```python
from build123d import *

# Parameters (mm, degrees)
F0_R     = 12.7
F1_DEPTH = 127
F2_R     = 3.175
F3_W     = 3.429
F3_H     = 3.429
F4_DEPTH = 127.001


with BuildPart() as f1:
    # F0 (on Top) → F1 (new body)
    with BuildSketch(Plane.XY):
        Circle(F0_R)
    extrude(amount=F1_DEPTH)

    # F2
    f2_edges = [f1.edges().sort_by_distance(p)[0] for p in [
        (-12.7, 0, 127),
    ]]
    fillet(f2_edges, radius=F2_R)

    # F3 (on face) → F4 (cut, through all)
    with BuildSketch(Plane.XY.offset(127)):
        Rectangle(F3_W, F3_H)
    extrude(amount=-F4_DEPTH, mode=Mode.SUBTRACT)


solid = f1.part
```
Geometry check sheet. Reference: the model listing, model coordinates, mm. A direction names the side the tool comes from. Give positions to 0.01 mm unless a question says otherwise; leave off trailing zeros. Write each loop counter-clockwise with the first axis right and the second up, starting at its lowest first coordinate (ties: lowest second). Pieces come first, ordered by that corner, then holes.
1) Gauge pin test, flat ends, axial feed: pin 1 (5 mm diameter, centred on x = -4, z = 93.5, fed in from -Y); pin 2 (8 mm diameter, centred on y = -5.5, z = 65.5, fed in from +X); pin 3 (1.5 mm diameter, centred on x = -0.5, y = 0, fed in from +Z); pin 4 (1 mm diameter, centred on x = -8.5, z = 25, fed in from +Y). Record the tip position at first contact, or that the pin passes through.
2) Access from +Z, -Z, +X, -X, +Y, -Y to the whole of each face (thin tool, end or side, straight path). Record for faces 5 (the flat face through (-1.714, 0, 64)), 6 (the flat face through (3, 0, 0)).
3) Material ranges on L1, parallel to Y at x = 0.75, z = 68; L2, parallel to Y at x = -1.25, z = 48.5; L3, parallel to X at y = 6, z = 113, recorded low to high.
4) Section check C-C, the plane z = 41.5. Record the boundary of the cut face in (x, y), and give its area (3 significant figures).
5) Release check for a two-part mould opening along X. For faces 1 (the flat face through (2, 0, 127)), 2 (the flat face through (0, 1.714, 64)), 3 (the cylindrical face through (-2.75, -12.4, 61.05)), 4 (the flat face through (1.714, 0, 64)) record: pulls with the +X half, pulls with the -X half, needs draft (parallel to the pull), parting line crosses it, or undercut.
Computed:
1. pin 1: stops at y = -12.61
1. pin 2: stops at x = 12.61
1. pin 3: passes through
1. pin 4: stops at y = 9.86
2. face 5: +Z, -Z
2. face 6: -Z, +X, -X, +Y, -Y
3. L1: y = -12.68 to -1.71, 1.71 to 12.68
3. L2: y = -12.64 to -1.71, 1.71 to 12.64
3. L3: x = -11.19 to 11.19
4. outline: circle Ø25.4 at (0, 0); hole (-1.71, -1.71) - (1.71, -1.71) - (1.71, 1.71) - (-1.71, 1.71) - close
4. area: 495 mm2
5. face 1: needs draft
5. face 2: undercut
5. face 3: parting line crosses it
5. face 4: undercut
